Geometry check sheet. Reference: the model listing, model coordinates, mm. A direction names the side the tool comes from. Round coordinates to 2 decimals unless told otherwise and drop trailing zeros. Order: outer loops, then holes, each group sorted by start corner. A loop starts at its lowest first (then second) coordinate and runs counter-clockwise, first axis right, second up. Notation, with made-up numbers: (87, 58.25) - (132, 58.25) arc R20 cw to (132, 92.25) - close; hole circle Ø3 at (61.5, 87.25). An arc over 180 degrees is marked (long way). Return JSON: item names as keys, results as strings. Group by question number.
Q1. Tool access check on faces 1 (the flat face through (0, 57, 30)), 2 (the flat face through (0, 71.906, 58)), 3 (the flat face through (0.21, 88.615, 49.72)), 4 (the flat face through (0, -15, 15)). Record the directions out of +Z, -Z, +X, -X, +Y, -Y that give a thin tool (end or side, any length) a straight path to the whole face; none if there is none.
Q2. Material ranges on line 1 along Z through (x, y) = (-7.5, -15.5); line 2 along Z through (x, y) = (-12.25, 72.5); line 3 along Y through (x, z) = (-7.5, 13.5), recorded low to high.
Q3. Draft check along Y on faces 5 (the flat face through (0, -71.906, 58)), 6 (the flat face through (0, -57, 30)), 7 (the flat face through (0.21, -88.615, 49.72)). Enter one of: pulls with the +Y half, pulls with the -Y half, needs draft (parallel to the pull), parting line crosses it, or undercut.
Q4. Sectioned sample at A-A, the plane x = -2.25. Record the cut outline in (y, z).
Q5. Sectioned sample at B-B, the plane z = 62.5. Record the cut outline in (x, y), then the cut area to 3 significant figures.
Q6. Sectioned sample at C-C, the plane y = -18. Record the cut outline in (x, z), then the cut area to 3 significant figures.
Q7. Gauge pin test, flat ends, axial feed: pin 1 Ø4 at (x, y) = (-9.5, 10) entering from +Z; pin 2 Ø6 at (x, z) = (5.5, 18) entering from +Y; pin 3 Ø4 at (x, y) = (10, 54.5) entering from -Z. Record the tip position at first contact, or that the pin passes through.
Q8. Sectioned sample at D-D, the plane z = 22. Record the cut outline in (x, y), then the cut area to 3 significant figures.
```python
from build123d import *

# Parameters (mm, degrees)
SKETCH1_W           = 30
SKETCH1_H           = 30
BOSS_EXTRUDE1_DEPTH = 30
BOSS_EXTRUDE2_DEPTH = 15


with BuildPart() as part:
    # Sketch1 → Boss-Extrude1 (new body)
    with BuildSketch(Plane.XY):
        Rectangle(SKETCH1_W, SKETCH1_H)
    extrude(amount=BOSS_EXTRUDE1_DEPTH)

    # Sketch2 → Boss-Extrude2 (add, symmetric)
    with BuildSketch(Plane(origin=(0, 0, 0), x_dir=(0, 0, -1), z_dir=(1, 0, 0))):
        Polygon((-30, 15), (-30, 100), (-70, 76.905989232), (-70, 71.905989232), (-45, 71.905989232), (-45, 0), (-30, 0), align=None)
    boss_extrude2 = extrude(amount=BOSS_EXTRUDE2_DEPTH, both=True)

    # Mirror1: Boss-Extrude2 across plane
    add(boss_extrude2.mirror(Plane.ZX))


solid = part.part
```
Reply:
{
 "1": {"face 1": "-Z, +X, -X, +Y", "face 2": "+Z, +X, -X", "face 3": "+Z, +X, -X, +Y", "face 4": "-Z, +X, -X, -Y"},
 "2": {"line 1": "30 to 45", "line 2": "30 to 70", "line 3": "-15 to 15"},
 "3": {"face 5": "undercut", "face 6": "needs draft", "face 7": "pulls with the -Y half"},
 "4": {"outline": "(-100, 30) - (-15, 30) - (-15, 0) - (15, 0) - (15, 30) - (100, 30) - (76.91, 70) - (71.91, 70) - (71.91, 45) - (-71.91, 45) - (-71.91, 70) - (-76.91, 70) - close"},
 "5": {"outline": "(-15, -81.24) - (15, -81.24) - (15, -71.91) - (-15, -71.91) - close; (-15, 71.91) - (15, 71.91) - (15, 81.24) - (-15, 81.24) - close", "area": "560 mm^2"},
 "6": {"outline": "(-15, 30) - (15, 30) - (15, 45) - (-15, 45) - close", "area": "450 mm^2"},
 "7": {"pin 1": "z = 45", "pin 2": "y = 15", "pin 3": "z = 30"},
 "8": {"outline": "(-15, -15) - (15, -15) - (15, 15) - (-15, 15) - close", "area": "900 mm^2"}
}
